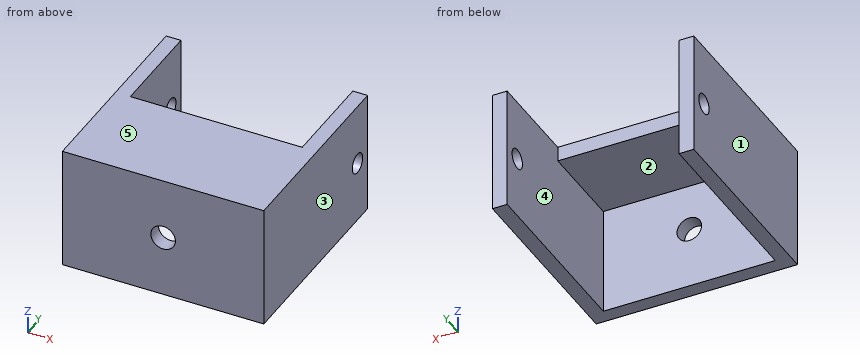
Autodesk Inventor part; units mm, degrees
ref_plane "YZ Plane" through (0, 0, 0) normal (1, 0, 0) x (0, 1, 0)
ref_plane "XZ Plane" through (0, 0, 0) normal (0, 1, 0) x (-1, 0, 0)
ref_plane "XY Plane" through (0, 0, 0) normal (0, 0, 1) x (1, 0, 0)
sketch "Sketch1" plane through (0, 0, 0) normal (0, 1, 0) x (-1, 0, 0)
  line L0 (130.175, 79.375) -> (-130.175, 79.375)
  line L1 (-130.175, 79.375) -> (-130.175, -79.375)
  line L2 (-130.175, -79.375) -> (130.175, -79.375)
  line L3 (130.175, -79.375) -> (130.175, 79.375)
  line L4 (130.175, 79.375) -> (-130.175, -79.375) construction
  line L5 (-130.175, 79.375) -> (130.175, -79.375) construction
  point P0 (0, 0)
  dimension "d0" = 260.35
  dimension "d1" = 158.75
extrude "Base" add sketch "Sketch1" against normal blind 19.05
sketch "Sketch2" plane through (0, 0, 0) normal (0, 1, 0) x (1, 0, 0)
  line L0 (-130.175, -79.375) -> (-130.175, 79.375)
  line L1 (-130.175, 79.375) -> (-111.125, 79.375)
  line L2 (-111.125, 79.375) -> (-111.125, -79.375)
  line L3 (-111.125, -79.375) -> (-130.175, -79.375)
  line L4 (-130.175, -79.375) -> (-130.175, 79.375)
  line L5 (130.175, 79.375) -> (130.175, -79.375)
  line L6 (130.175, -79.375) -> (-130.175, -79.375)
  line L7 (130.175, 79.375) -> (111.125, 79.375)
  line L8 (111.125, 79.375) -> (111.125, -79.375)
  line L9 (111.125, -79.375) -> (130.175, -79.375)
  line L10 (130.175, -79.375) -> (130.175, 79.375)
  line L11 (-130.175, -79.375) -> (130.175, -79.375)
  point P0 (0, 0)
  dimension "d4" = 19.05
extrude "Sides" add sketch "Sketch2" along normal blind 241.3
sketch "Sketch3" plane through (0, 0, 0) normal (0, 1, 0) x (1, 0, 0)
  line L0 (-130.175, -79.375) -> (-111.125, -79.375)
  line L1 (111.125, 79.375) -> (111.125, -79.375)
  line L2 (-111.125, -79.375) -> (111.125, -79.375)
  line L3 (111.125, -79.375) -> (111.125, -60.325)
  line L4 (111.125, -60.325) -> (-111.125, -60.325)
  line L5 (-111.125, -60.325) -> (-111.125, -79.375)
  point P0 (0, 0)
  point P1 (111.125, -79.375)
  dimension "d7" = 19.05
extrude "FrontPiece" add sketch "Sketch3" along normal blind 114.3
sketch "Sketch5" plane through (130.175, -19.05, 79.375) normal (1, 0, 0) x (0, 0, -1)
  line L0 (158.75, 260.35) -> (0, 260.35) construction
  line L1 (79.375, 260.35) -> (79.375, 0) construction
  line L2 (0, 0) -> (158.75, 0) construction
  line L3 (19.05, 19.05) -> (158.75, 19.05)
  point P0 (79.375, 19.05)
  point P1 (79.375, 234.95)
  dimension "d23" = 215.9
hole "HoleForSides" at (130.175, 215.9, 0) direction (-1, 0, 0) diameter 25.908 end through all
sketch "Sketch8" plane through (0, 0, 0) normal (0, 1, 0) x (1, 0, 0)
  circle A0 centre (0, 0) radius 15.875
  dimension "d27" = 31.75
extrude "BottomHole" cut sketch "Sketch8" against normal through all
equation "\"d0\" = interiorWidth + 2 * woodThickness"
equation "\"d1\" = partDepth"
equation "\"d2\" = woodThickness"
equation "\"d4\" = woodThickness"
equation "\"d5\" = totalHeight - woodThickness"
equation "\"d7\" = woodThickness"
equation "\"d8\" = supportBoardHeight"
equation "\"d13\" = holeDiameter"
equation "\"interiorWidth\" = 222.25"
equation "\"woodThickness\" = 19.05"
equation "\"holeCenter\" = 215.9"
equation "\"supportBoardHeight\" = 114.3"
equation "\"holeDiameter\" = 25.908"
equation "\"partDepth\" = 158.75"
properties part number "woodForkAssembly02" material "Wood (Birch)"
Design review of the part built by this model. Coordinates are the model's own, in mm. Face numbers are marked on the shaded views. A direction names the side the tool comes from. Round coordinates to 2 decimals unless told otherwise and drop trailing zeros. Loops run counter-clockwise (first coordinate to the right, second up) from the corner with the lowest first, then second, coordinate; pieces in that order, holes last. Notation, with made-up numbers: (34, -5) - (68, -5) arc R17 cw to (68, 12) - close; hole circle Ø11 at (66, -30.5). An arc over 180 degrees is marked (long way). One line per question, with ' | ' between items.
1. For L1, parallel to X at y = 122, z = -67.5 (3 decimals); L2, parallel to Z at x = 0, y = -10.25 (3 decimals); L3, parallel to Z at x = 117.5, y = 215.9 (3 decimals), list the stretches that pass through material, from the lowest coordinate up. Write a range as [from, to].
Results are:
L1: x = [-130.175, -111.125], [111.125, 130.175] | L2: z = [-79.375, -15.875], [15.875, 79.375] | L3: z = [-79.375, -12.954], [12.954, 79.375]
2. We need section C-C, the plane x = 0. State the section outline as (y, z) points (3 decimals), and give its area (3 significant figures).
Results are:
outline: (-19.05, -79.375) - (0, -79.375) - (0, -15.875) - (-19.05, -15.875) - close; (-19.05, 15.875) - (0, 15.875) - (0, 60.325) - (114.3, 60.325) - (114.3, 79.375) - (-19.05, 79.375) - close | area: 4,600 mm²
3. Draft analysis for pull direction X (two halves, no side actions). For the marked faces 3, 4 and 5, state which applies: released by +X, released by -X, zero draft, split by the parting line, or undercut.
Results are:
face 3: released by +X | face 4: undercut | face 5: zero draft
4. We need section B-B, the plane y = 215.9. State the section outline as (x, z) points (3 decimals).
Results are:
outline: (-130.175, -79.375) - (-111.125, -79.375) - (-111.125, -12.954) - (-130.175, -12.954) - close; (-130.175, 12.954) - (-111.125, 12.954) - (-111.125, 79.375) - (-130.175, 79.375) - close; (111.125, -79.375) - (130.175, -79.375) - (130.175, -12.954) - (111.125, -12.954) - close; (111.125, 12.954) - (130.175, 12.954) - (130.175, 79.375) - (111.125, 79.375) - close
5. We need section A-A, the plane z = 0. State the section outline as (x, y) points (3 decimals).
Results are:
outline: (-130.175, -19.05) - (-15.875, -19.05) - (-15.875, 0) - (-111.125, 0) - (-111.125, 202.946) - (-130.175, 202.946) - close; (-130.175, 228.854) - (-111.125, 228.854) - (-111.125, 241.3) - (-130.175, 241.3) - close; (15.875, -19.05) - (130.175, -19.05) - (130.175, 202.946) - (111.125, 202.946) - (111.125, 0) - (15.875, 0) - close; (111.125, 228.854) - (130.175, 228.854) - (130.175, 241.3) - (111.125, 241.3) - close
6. We need section D-D, the plane y = 143.5. State the section outline as (x, z) points (3 decimals).
Results are:
outline: (-130.175, -79.375) - (-111.125, -79.375) - (-111.125, 79.375) - (-130.175, 79.375) - close; (111.125, -79.375) - (130.175, -79.375) - (130.175, 79.375) - (111.125, 79.375) - close
7. Clearance check with flat-ended pins moving along their axes: P1, Ø5.5, axis at x = 40.5, z = 68.5, coming from the +Y side; P2, Ø3, axis at x = 88, z = -3, coming from the +Y side; P3, Ø1, axis at x = 46, y = 84, coming from the -Z side (3 decimals); P4, Ø20.5, axis at y = 215.9, z = 0, coming from the +X side. State where each tip first meets the part, or that it passes through.
Results are:
P1: stops at y = 114.3 | P2: stops at y = 0 | P3: stops at z = 60.325 | P4: passes through
8. For the marked faces 1 and 2, list the 3-axis set-ups (+Z, -Z, +X, -X, +Y, -Y) from which the entire face can be reached by the end or side of a thin tool; tool diameter is ignored.
Results are:
face 1: +Z, -Z, -X, +Y, -Y | face 2: -Z, +Y
